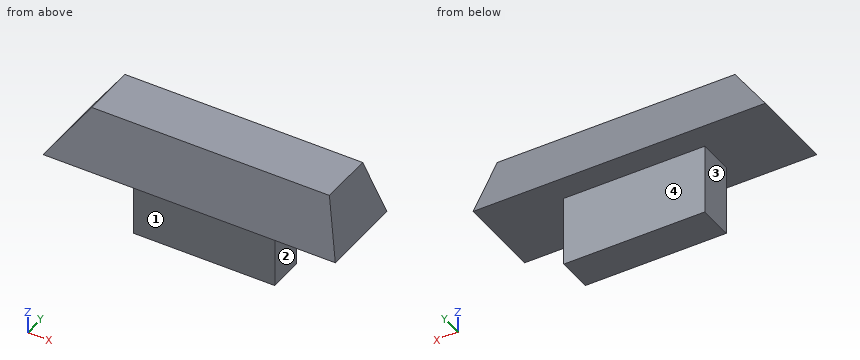
```python
from build123d import *

# Parameters (mm, degrees)
SKETCH1_W           = 13.155170484
SKETCH1_H           = 3.81
BOSS_EXTRUDE1_DEPTH = 2.54
CHAMFER1_SIZE       = 2.54
CHAMFER1_SIZE_2     = 1.778527147
CHAMFER2_SIZE       = 0.680590949
CHAMFER2_SIZE_2     = 2.54
SKETCH2_W           = 6.35
SKETCH2_H           = 1.5875
BOSS_EXTRUDE3_DEPTH = 3.175


with BuildPart() as part:
    # Sketch1 → Boss-Extrude1 (new body)
    with BuildSketch(Plane.XY):
        with Locations((76.924914758, 65.532)):
            Rectangle(SKETCH1_W, SKETCH1_H)
    extrude(amount=BOSS_EXTRUDE1_DEPTH)

    # Chamfer1
    # the kernel refuses this chamfer: 2.54, 1.778527147 mm, written as the material it takes off along each edge
    with BuildSketch(Plane(origin=(70.347329516, 73.996682665, 2.54), x_dir=(-0.02220967419845826, 0, -0.9997533347641299), z_dir=(0, -1, 0))) as chamfer1_piece_1:
        Polygon((CHAMFER1_SIZE * 0.999753334764, CHAMFER1_SIZE * 0.0222096741985), (-CHAMFER1_SIZE_2 * 0.0222096741991, CHAMFER1_SIZE_2 * 0.999753334794), (0, 0), align=None)
    extrude(amount=16.92936533, mode=Mode.SUBTRACT)

    # Chamfer2
    # the kernel refuses this chamfer: 2.54, 0.680590949 mm, written as the material it takes off along each edge
    with BuildSketch(Plane(origin=(65.530183875, 63.627, 2.54), x_dir=(0, 0.9905000388259545, 0.13751244702128823), z_dir=(1, 0, 0))) as chamfer2_piece_1:
        Polygon((CHAMFER2_SIZE * 0.990500038499, -CHAMFER2_SIZE * 0.137512446976), (-CHAMFER2_SIZE_2 * 0.137512447021, -CHAMFER2_SIZE_2 * 0.990500038826), (0, 0), align=None)
    extrude(amount=24.567988913, mode=Mode.SUBTRACT)
    with BuildSketch(Plane(origin=(83.5025, 57.031327212, 2.54), x_dir=(-0.9905000388259543, 0, 0.13751244702128956), z_dir=(0, 1, 0))) as chamfer2_piece_2:
        Polygon((CHAMFER2_SIZE * 0.990500038499, -CHAMFER2_SIZE * 0.137512446976), (-CHAMFER2_SIZE_2 * 0.137512447021, -CHAMFER2_SIZE_2 * 0.990500038826), (0, 0), align=None)
    extrude(amount=17.001345577, mode=Mode.SUBTRACT)
    with BuildSketch(Plane(origin=(90.098172788, 67.437, 2.54), x_dir=(0, 0.009967146577158238, -0.9999503267608394), z_dir=(-1, 0, 0))) as chamfer2_piece_3:
        Polygon((CHAMFER2_SIZE_2 * 0.999950326761, CHAMFER2_SIZE_2 * 0.00996714657716), (-CHAMFER2_SIZE * 0.00996714657386, CHAMFER2_SIZE * 0.99995032643), (0, 0), align=None)
    extrude(amount=24.567988913, mode=Mode.SUBTRACT)

    # Sketch2 → Boss-Extrude3 (add)
    with BuildSketch(Plane(origin=(0, 0, 0), x_dir=(-1, 0, 0), z_dir=(0, 0, -1))):
        with Locations((-76.924914758, 65.532)):
            Rectangle(SKETCH2_W, SKETCH2_H)
    extrude(amount=BOSS_EXTRUDE3_DEPTH)


solid = part.part
```
Build history of the part. All positions in model axes, mm. Face numbers are marked on the shaded views. A direction names the side the tool comes from. Coordinates: 2 decimals unless noted, no trailing zeros. Write each loop counter-clockwise with the first axis right and the second up, starting at its lowest first coordinate (ties: lowest second). Pieces come first, ordered by that corner, then holes.
1. Band-saw the part on B-B, the plane x = 77.5. Give the cut face in (y, z) (3 decimals), and give its area (3 significant figures).
Answer block:
outline: (63.627, 0) - (64.738, 0) - (64.738, -3.175) - (66.326, -3.175) - (66.326, 0) - (67.437, 0) - (66.756, 2.54) - (64.308, 2.54) - close
area: 13.0 mm2
2. Drop flat-ended pins along their axis: pin 1 (1.7 mm diameter, centred on y = 65.5, z = -1, fed in from -X); pin 2 (1.7 mm diameter, centred on y = 65.5, z = -1, fed in from +X). Give the stop position or say it passes through.
Answer block:
pin 1: stops at x = 73.75
pin 2: stops at x = 80.1
3. Band-saw the part on C-C, the plane z = -1.5. Give the cut face in (x, y).
Answer block:
outline: (73.75, 64.74) - (80.1, 64.74) - (80.1, 66.33) - (73.75, 66.33) - close
4. Drill centre lines: probe 1 along X at (y, z) = (65.95, -2.45); probe 2 along Z at (x, y) = (73.5, 65.35); probe 3 along Y at (x, z) = (79.25, -0.75). Where is each one in solid material? Low to high.
Answer block:
probe 1: x = 73.75 to 80.1
probe 2: z = 0 to 2.54
probe 3: y = 64.74 to 66.33
5. 3-axis set-ups, long thin cutter, end or side, ignore diameter. For the marked faces 1, 2, 3 and 4: which of +Z, -Z, +X, -X, +Y, -Y reach the whole face in a straight line?
Answer block:
face 1: -Z, +X, -X, -Y
face 2: -Z, +X, +Y, -Y
face 3: -Z, -X, +Y, -Y
face 4: -Z, +X, -X, +Y
6. Band-saw the part on D-D, the plane x = 72.75. Give the cut face in (y, z), and give its area (3 significant figures).
Answer block:
outline: (63.63, 0) - (67.44, 0) - (66.76, 2.54) - (64.31, 2.54) - close
area: 7.95 mm2
7. Band-saw the part on A-A, the plane y = 65.4. Give the cut face in (x, z) (1 decimal).
Answer block:
outline: (70.3, 0) - (73.7, 0) - (73.7, -3.2) - (80.1, -3.2) - (80.1, 0) - (83.5, 0) - (82.8, 2.5) - (72.1, 2.5) - close
